from build123d import *

# Parameters (mm, degrees)
SKETCH_1_R      = 5
SKETCH_1_W      = 5.5
SKETCH_1_H      = 5.5
EXTRUDE_1_DEPTH = 2.5
SKETCH_3_R      = 5
SKETCH_3_W      = 3.5
SKETCH_3_H      = 3.5
EXTRUDE_3_DEPTH = 0.5


with BuildPart() as part:
    # 草图1 → 凸台-拉伸1 (new body)
    with BuildSketch(Plane(origin=(0, 0, 0), x_dir=(0, 0, -1), z_dir=(1, 0, 0))):
        Circle(SKETCH_1_R)
        Rectangle(SKETCH_1_W, SKETCH_1_H, mode=Mode.SUBTRACT)
    extrude(amount=EXTRUDE_1_DEPTH)

    # 草图3 → 凸台-拉伸3 (add)
    with BuildSketch(Plane(origin=(2.5, 0, 0), x_dir=(0, 0, -1), z_dir=(1, 0, 0))):
        Circle(SKETCH_3_R)
        Rectangle(SKETCH_3_W, SKETCH_3_H, mode=Mode.SUBTRACT)
    extrude(amount=EXTRUDE_3_DEPTH)


solid = part.part
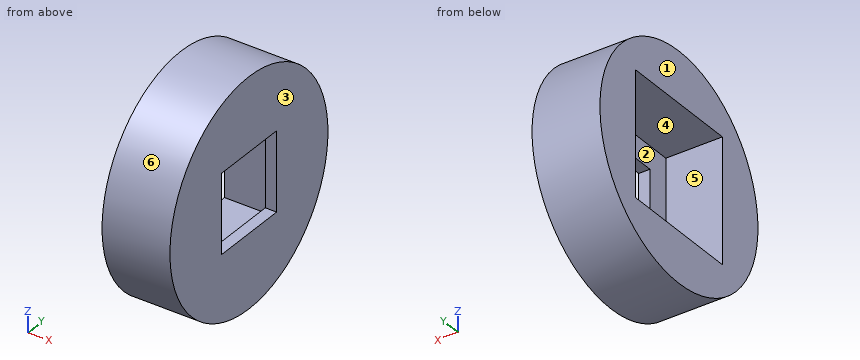
Geometry: final body of the model. Coordinates: model frame, mm. Face numbers are marked on the shaded views. A direction names the side the tool comes from. Give positions to 0.01 mm unless a question says otherwise; leave off trailing zeros. Write each loop counter-clockwise with the first axis right and the second up, starting at its lowest first coordinate (ties: lowest second). Pieces come first, ordered by that corner, then holes. Notation, with made-up numbers: (78, -10.5) - (116, -10.5) arc R21 cw to (116, 27.5) - close; hole circle Ø1 at (-20, 78). An arc over 180 degrees is marked (long way). Return JSON: item names as keys, results as strings. Group by question number.
1) Section A-A on y = 0. Return the cut outline in (x, z), plus the area to 3 significant figures.
2) First-contact query: P1, Ø1.2, axis at x = 2, z = 1, coming from the +Y side; P2, Ø1.5, axis at x = 1, z = 1, coming from the -Y side; P3, Ø0.6, axis at x = 3, y = 0.5, coming from the +Z side. Flat tips, straight axial feed; report the tip coordinate or a pass-through.
3) Set-up query: the marked faces 1 and 2. Return all of +Z, -Z, +X, -X, +Y, -Y with unobstructed straight access to the full face (end or side cutting, diameter ignored); none if empty.
4) Section D-D on z = -4. Return the cut outline in (x, y).
5) Section C-C on x = 2.7. Return the cut outline in (y, z).
6) Line query: line 1 (Y direction, x = 2.6, z = 0); line 2 (X direction, y = 1.5, z = 2.25); line 3 (Z direction, x = 1.65, y = 1). Output: solid intervals per line, ascending.
7) Mould query, pull axis Y, two halves, no side actions, for the marked faces 3, 4, 5 and 6. Classes: released by +Y, released by -Y, zero draft, split by the parting line, or undercut.
Filled in:
{
 "1": {"outline": "(0, -5) - (3, -5) - (3, -1.75) - (2.5, -1.75) - (2.5, -2.75) - (0, -2.75) - close; (0, 2.75) - (2.5, 2.75) - (2.5, 1.75) - (3, 1.75) - (3, 5) - (0, 5) - close", "area": "14.5 mm^2"},
 "2": {"P1": "stops at y = 4.98", "P2": "stops at y = -4.99", "P3": "stops at z = 5"},
 "3": {"face 1": "+Z, -Z, -X, +Y, -Y", "face 2": "-X"},
 "4": {"outline": "(0, -3) - (3, -3) - (3, 3) - (0, 3) - close"},
 "5": {"outline": "circle Ø10 at (0, 0); hole (-1.75, -1.75) - (1.75, -1.75) - (1.75, 1.75) - (-1.75, 1.75) - close"},
 "6": {"line 1": "y = -5 to -1.75, 1.75 to 5", "line 2": "x = 2.5 to 3", "line 3": "z = -4.9 to -2.75, 2.75 to 4.9"},
 "7": {"face 3": "zero draft", "face 4": "undercut", "face 5": "undercut", "face 6": "split by the parting line"}
}
